from build123d import *

# Parameters (mm, degrees)
BOSS_EXTRUDE1_DEPTH      = 10
BOSS_EXTRUDE2_START      = -19.5635
BOSS_EXTRUDE2_DEPTH      = 39.127
M3_CLEARANCE_HOLE1_D     = 3.4
M3_CLEARANCE_HOLE1_DEPTH = 7.5
M3_CLEARANCE_HOLE1_TIP   = 1.021463052
M4_CLEARANCE_HOLE1_D     = 4.5
BOSS_EXTRUDE3_DEPTH      = 3


with BuildPart() as part:
    # Sketch1 → Boss-Extrude1 (new, symmetric)
    with BuildSketch(Plane.XY):
        Polygon((-19.5635, 0), (19.5635, 0), (19.5635, -31), (33.5635, -31), (33.5635, -27), (23.5635, -27), (23.5635, 4), (-23.5635, 4), (-23.5635, -27), (-33.5635, -27), (-33.5635, -31), (-19.5635, -31), align=None)
    extrude(amount=BOSS_EXTRUDE1_DEPTH, both=True)

    # Sketch2 → Boss-Extrude2 (add)
    with BuildSketch(Plane(origin=(0, 0, 0), x_dir=(0, 0, -1), z_dir=(1, 0, 0)).offset(BOSS_EXTRUDE2_START)):
        with BuildLine():
            Line((5e-09, 0), (-10, 0))
            Line((-10, 0), (-10, -3.581906476))
            ThreePointArc((-10, -3.581906476), (-5.311074607, -0.922492235), (5e-09, 0))
        make_face()
        with BuildLine():
            Line((10, 0), (5e-09, 0))
            ThreePointArc((5e-09, 0), (5.311074611, -0.922492237), (10, -3.581906476))
            Line((10, -3.581906476), (10, 0))
        make_face()
    extrude(amount=BOSS_EXTRUDE2_DEPTH)

    # M3 Clearance Hole1
    with Locations(Plane(origin=(0, -27, 0), x_dir=(1, 0, 0), z_dir=(0, 1, 0))):
        with Locations((28.5635, 0), (-28.5635, 0)):
            Hole(M3_CLEARANCE_HOLE1_D / 2, depth=M3_CLEARANCE_HOLE1_DEPTH)
            with Locations((0, 0, -(M3_CLEARANCE_HOLE1_DEPTH + M3_CLEARANCE_HOLE1_TIP / 2))):  # 118° drill point
                Cone(0, M3_CLEARANCE_HOLE1_D / 2, M3_CLEARANCE_HOLE1_TIP, mode=Mode.SUBTRACT)

    # M4 Clearance Hole1 (through all)
    with Locations(Plane(origin=(0, 4, 0), x_dir=(1, 0, 0), z_dir=(0, 1, 0))):
        with Locations((7.5635, 0)):
            Hole(M4_CLEARANCE_HOLE1_D / 2)

    # Sketch7 → Boss-Extrude3 (add)
    with BuildSketch(Plane.ZY.offset(23.5635)):
        Polygon((-10, 4), (-10, 5.5), (-6, 9.5), (-6, 4), align=None)
        with BuildLine():
            Line((-10, 6.207106781), (-6, 10.207106781))
            ThreePointArc((-6, 10.207106781), (0, 16.207106781), (6, 10.207106781))
            Line((6, 10.207106781), (6, 4))
            Line((6, 4), (10, 4))
            Line((10, 4), (10, 10.207106781))
            ThreePointArc((10, 10.207106781), (0, 20.207106781), (-10, 10.207106781))
            Line((-10, 10.207106781), (-10, 6.207106781))
        make_face()
    extrude(amount=-BOSS_EXTRUDE3_DEPTH)


solid = part.part
Can you work these out from the model? Positions are in its coordinate system, mm. A direction names the side the tool comes from. Coordinates: 2 decimals unless noted, no trailing zeros. Order: outer loops, then holes, each group sorted by start corner. A loop starts at its lowest first (then second) coordinate and runs counter-clockwise, first axis right, second up. Notation, with made-up numbers: M 0,-19.5 L 39,-19.5 A7 ccw 39,-8.5 Z; hole C 57.25,-23 d11. An arc over 180 degrees is marked long. Answer as CSV lines item,"result".
(1) Suppose I cut it at B-B on x = 8. Please give me the cut outline in (y, z), plus the area to 3 significant figures.
Geometry check:
outline,"M -3.58,-10 L 4,-10 L 4,-2.21 L -0.16,-2.21 A15.75 cw Z; M -3.58,10 A15.75 cw -0.16,2.21 L 4,2.21 L 4,10 Z"
area,"84.8 mm^2"
(2) Suppose I cut it at C-C on y = 13.5. Please give me the cut outline in (x, z).
Geometry check:
outline,"M -23.56,-9.44 L -20.56,-9.44 L -20.56,-5.02 L -23.56,-5.02 Z; M -23.56,5.02 L -20.56,5.02 L -20.56,9.44 L -23.56,9.44 Z"
(3) On a 3-axis mill with a long thin cutter (end or side, diameter ignored), from which of +Z, -Z, +X, -X, +Y, -Y can I reach the whole of each face in a straight line? I mean faces 1 (the cylindrical face through (-22.085, 16.206, -0.132)), 2 (the flat face through (-20.564, 6, -8)), 3 (the cylindrical face through (5.42, 1.89, -0.68)), 4 (the flat face through (-23.564, -8, 0)). Say none if no direction works.
Geometry check:
face 1,"+X, -X"
face 2,"+Z, -Z, +X, +Y"
face 3,"+Y, -Y"
face 4,"+Z, -Z, -X, +Y"
(4) If we mould it in two halves opening along Z, with no side actions, what happens to faces 5 (the cylindrical face through (-22.085, 20.205, 0.22)), 6 (the flat face through (-22.1, 7.5, -8)), 7 (the flat face through (-26.7, -31, 0.1))? For each: released by +Z, released by -Z, zero draft, split by the parting line, or undercut.
Geometry check:
face 5,"split by the parting line"
face 6,"undercut"
face 7,"zero draft"
(5) Suppose I cut it at D-D on y = 7. Please give me the cut outline in (x, z), plus the area to 3 significant figures.
Geometry check:
outline,"M -23.56,-10 L -20.56,-10 L -20.56,-9.21 L -23.56,-9.21 Z; M -23.56,-8.5 L -20.56,-8.5 L -20.56,-6 L -23.56,-6 Z; M -23.56,6 L -20.56,6 L -20.56,10 L -23.56,10 Z"
area,"21.9 mm^2"
(6) Suppose I cut it at A-A on z = -3. Please give me the cut outline in (x, y), plus the area to 3 significant figures.
Geometry check:
outline,"M -33.56,-31 L -19.56,-31 L -19.56,-0.29 L 19.56,-0.29 L 19.56,-31 L 33.56,-31 L 33.56,-27 L 23.56,-27 L 23.56,4 L -23.56,4 L -23.56,-27 L -33.56,-27 Z; M -23.56,15.4 L -20.56,15.4 L -20.56,19.75 L -23.56,19.75 Z"
area,"541 mm^2"
(7) Please list where these lines run through material, in increasing order: L1, parallel to X at y = 2.5, z = 0; L2, parallel to X at y = -27.5, z = -8.25; L3, parallel to Y at x = -20.5, z = -0.5.
Geometry check:
L1,"-23.56 to 5.31, 9.81 to 23.56"
L2,"-33.56 to -19.56, 19.56 to 33.56"
L3,"-31 to 4"
(8) I'm going to push flat-ended pins straight in: pin 1 (3 mm diameter, centred on y = 8, z = -8, fed in from +X); pin 2 (3 mm diameter, centred on x = 22, z = 7.5, fed in from +Y); pin 3 (5 mm diameter, centred on x = -28, z = -2.5, fed in from +Y). Where does each tip first touch, or does it pass through?
Geometry check:
pin 1,"x = -20.56"
pin 2,"y = 4"
pin 3,"y = -27"
